from build123d import *

# Parameters (mm, degrees)
BOSS_EXTRUDE1_DEPTH = 14
SKETCH5_OUTSIDE_W   = 36.988
SKETCH5_OUTSIDE_H   = 125.051
CUT_EXTRUDE1_DEPTH  = 100.116594104


with BuildPart() as part:
    # Sketch2 → Boss-Extrude1 (new body)
    with BuildSketch(Plane(origin=(0, 0, 0), x_dir=(0, 0, -1), z_dir=(1, 0, 0))):
        with BuildLine():
            ThreePointArc((6, 0), (0, 6), (-6, 0))
            Line((-6, 0), (-9.742143433, -32.743755036))
            ThreePointArc((-9.742143433, -32.743755036), (0, -25), (9.742143433, -32.743755036))
            Line((9.742143433, -32.743755036), (6, 0))
        make_face()
        with BuildLine():
            ThreePointArc((9.742143433, -32.743755036), (0, -25), (-9.742143433, -32.743755036))
            Line((-9.742143433, -32.743755036), (-10, -35))
            Line((-10, -35), (-4, -35))
            ThreePointArc((-4, -35), (0, -31), (4, -35))
            Line((4, -35), (10, -35))
            Line((10, -35), (9.742143433, -32.743755036))
        make_face()
        with BuildLine():
            Line((-4, -35), (-10, -35))
            ThreePointArc((-10, -35), (-8.730548592, -39.876219979), (-5.244495744, -43.514415094))
            Line((-5.244495744, -43.514415094), (10, -35))
            Line((10, -35), (4, -35))
            ThreePointArc((4, -35), (0, -39), (-4, -35))
        make_face()
        with BuildLine():
            Line((10, -57), (10, -35))
            ThreePointArc((10, -35), (5.587707823, -43.293221406), (-3.755504256, -44.268019626))
            ThreePointArc((-3.755504256, -44.268019626), (-0.269451408, -47.906214741), (1, -52.78243472))
            Line((1, -52.78243472), (1, -57))
            Line((1, -57), (5.433108836, -88.085634368))
            ThreePointArc((5.433108836, -88.085634368), (4.995673886, -89.718617368), (3.463525492, -90.433113071))
            Line((3.463525492, -90.433113071), (-1.036474508, -90.433113071))
            ThreePointArc((-1.036474508, -90.433113071), (-2.926584774, -91.396172354), (-1.963525492, -93.28628262))
            Line((-1.963525492, -93.28628262), (6.388437813, -96))
            ThreePointArc((6.388437813, -96), (8.892790723, -95.390514833), (10, -93.062996137))
            Line((10, -93.062996137), (10, -57))
        make_face()
        with BuildLine():
            Line((10, -35), (-5.244495744, -43.514415094))
            ThreePointArc((-5.244495744, -43.514415094), (-4.484252006, -43.860102062), (-3.755504256, -44.268019626))
            ThreePointArc((-3.755504256, -44.268019626), (5.587707823, -43.293221406), (10, -35))
        make_face()
    extrude(amount=BOSS_EXTRUDE1_DEPTH)

    # Sketch5 outside → Cut-Extrude1 (cut, through all)
    with BuildSketch(Plane(origin=(0, 0, -10), x_dir=(-1, 0, 0), z_dir=(0, 0, -1))):
        with Locations((-7, -45.0315)):
            Rectangle(SKETCH5_OUTSIDE_W, SKETCH5_OUTSIDE_H)
        Polygon((0, -96.062996137), (-14, -96.062996137), (-9.5, -35), (-9.5, 6), (-4.5, 6), (-4.5, -35), align=None, mode=Mode.SUBTRACT)
    extrude(amount=-CUT_EXTRUDE1_DEPTH, mode=Mode.SUBTRACT)


solid = part.part
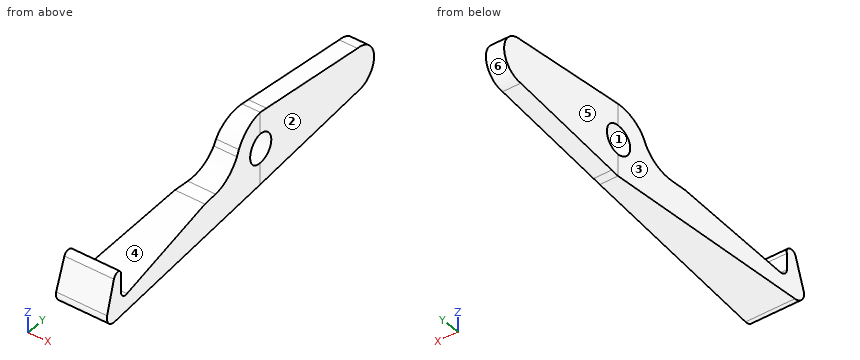
Part model, mm, in its own coordinate system. Face numbers are marked on the shaded views. A direction names the side the tool comes from. Coordinates: 2 decimals unless noted, no trailing zeros. Loops run counter-clockwise (first coordinate to the right, second up) from the corner with the lowest first, then second, coordinate; pieces in that order, holes last. Notation, with made-up numbers: (24.5, -26) -> (47.5, -26) arc R22 cw to (47.5, -18) -> close; hole circle Ø7 at (76, 66). An arc over 180 degrees is marked (long way). Use a Markdown table: item, result. Add a question column.
Item 1: Pull direction Y, two halves, no side cores. Call the marked faces 1, 2 and 3: +Y half, -Y half, draft (parallel to the pull), parting line (faces both ways), or undercut.
Item 2: Band-saw the part on A-A on x = 6.25. Write the cut outline in (y, z), plus the area to 3 significant figures.
Item 3: Band-saw the part on D-D on y = -23.5. Write the cut outline in (x, z), plus the area to 3 significant figures.
Item 4: Band-saw the part on C-C on y = -49.5. Write the cut outline in (x, z), plus the area to 3 significant figures.
Item 5: Flat gauge pins, fed straight in: P1, Ø6, axis at y = -62.5, z = -6.5, coming from the -X side; P2, Ø5, axis at y = -40, z = -4.5, coming from the +X side; P3, Ø10.5, axis at y = -35, z = 0, coming from the +X side. Where does each tip first touch, or does it go through?
Item 6: Band-saw the part on B-B on z = 0. Write the cut outline in (x, y), plus the area to 3 significant figures.
Item 7: Probe probe 1 along Z at (x, y) = (5.55, -35); probe 2 along Y at (x, z) = (7.6, 0); probe 3 along X at (y, z) = (-57, -1.25). List the from-to ranges inside material, lowest first.
Item 8: Which spindle directions (+Z, -Z, +X, -X, +Y, -Y) get a long thin tool onto all of the face, cutting with end or side? Do the marked faces 4, 5 and 6. Say none if no direction does.
Geometry says:
| question | item | result |
|---|---|---|
| 1 | face 1 | undercut |
| 1 | face 2 | draft |
| 1 | face 3 | +Y half |
| 2 | outline | (-96, -6.39) arc R3 ccw to (-93.06, -10) -> (-35, -10) -> (0, -6) arc R6 ccw to (0, 6) -> (-35, 10) arc R10 ccw to (-43.51, 5.24) arc R10 cw to (-52.78, -1) -> (-57, -1) -> (-88.09, -5.43) arc R2 cw to (-90.43, -3.46) -> (-90.43, 1.04) arc R1.5 ccw to (-93.29, 1.96) -> close; hole circle Ø8 at (-35, 0) |
| 2 | area | 1,140 mm² |
| 3 | outline | (4.5, -8.69) -> (9.5, -8.69) -> (9.5, 8.69) -> (4.5, 8.69) -> close |
| 3 | area | 86.9 mm² |
| 4 | outline | (3.43, -10) -> (10.57, -10) -> (10.57, -0.45) -> (3.43, -0.45) -> close |
| 4 | area | 68.2 mm² |
| 5 | P1 | x = 2.25 |
| 5 | P2 | x = 10.05 |
| 5 | P3 | x = 9.89 |
| 6 | outline | (0.16, -93.92) -> (13.84, -93.92) -> (13.59, -90.43) -> (0.41, -90.43) -> close; (3.51, -48.42) -> (10.49, -48.42) -> (9.79, -39) -> (4.21, -39) -> close; (4.5, -31) -> (9.5, -31) -> (9.5, 6) -> (4.5, 6) -> close |
| 6 | area | 291 mm² |
| 7 | probe 1 | -10 to -4, 4 to 10 |
| 7 | probe 2 | -93.92 to -90.43, -48.42 to -39, -31 to 6 |
| 7 | probe 3 | 2.88 to 11.12 |
| 8 | face 4 | +Z, +X, -X |
| 8 | face 5 | +Z, -Z, -X, +Y |
| 8 | face 6 | +X, -X, +Y |
